Input: part model. Units: mm. Frame: model coordinates. Give positions to 0.01 mm unless a question says otherwise; leave off trailing zeros. Order: outer loops, then holes, each group sorted by start corner. A loop starts at its lowest first (then second) coordinate and runs counter-clockwise, first axis right, second up.
```python
from build123d import *

# Parameters (mm, degrees)
SKETCH2_W           = 50
SKETCH2_H           = 50
BOSS_EXTRUDE1_DEPTH = 5
SKETCH6_W           = 42.36475395
SKETCH6_H           = 2.5
CUT_EXTRUDE1_DEPTH  = 50
SKETCH9_W           = 1.188642814
SKETCH9_H           = 2.221510963
CUT_EXTRUDE3_DEPTH  = 50
FILLET2_R           = 1
FILLET3_R           = 1
SKETCH11_W          = 1.18864281
SKETCH11_H          = 2.22151096
CUT_EXTRUDE4_DEPTH  = 50
FILLET5_R           = 1
FILLET6_R           = 1
SKETCH14_W          = 3.817623025
SKETCH14_H          = 0.21818248
CUT_EXTRUDE5_DEPTH  = 50
SKETCH16_W          = 3.817623025
SKETCH16_H          = 0.211754728
CUT_EXTRUDE6_DEPTH  = 50


with BuildPart() as part:
    # Sketch2 → Boss-Extrude1 (new body)
    with BuildSketch(Plane(origin=(0, 0, 0), x_dir=(1, 0, 0), z_dir=(0, 1, 0))):
        Rectangle(SKETCH2_W, SKETCH2_H)
    extrude(amount=BOSS_EXTRUDE1_DEPTH)

    # Sketch6 → Cut-Extrude1 (cut)
    with BuildSketch(Plane(origin=(0, 0, -25), x_dir=(-1, 0, 0), z_dir=(0, 0, -1))):
        with Locations((0, 1.25)):
            Rectangle(SKETCH6_W, SKETCH6_H)
    extrude(amount=-CUT_EXTRUDE1_DEPTH, mode=Mode.SUBTRACT)

    # Sketch9 → Cut-Extrude3 (cut)
    with BuildSketch(Plane(origin=(0, 0, -25), x_dir=(-1, 0, 0), z_dir=(0, 0, -1))):
        with Locations((-21.776698382, 1.389244518)):
            Rectangle(SKETCH9_W, SKETCH9_H)
    extrude(amount=-CUT_EXTRUDE3_DEPTH, mode=Mode.SUBTRACT)

    # Fillet2
    fillet2_edges = [part.edges().sort_by_distance(p)[0] for p in [
        (22.371019789, 2.5, 0),
    ]]
    fillet(fillet2_edges, radius=FILLET2_R)

    # Fillet3
    fillet3_edges = [part.edges().sort_by_distance(p)[0] for p in [
        (22.371019789, 0.278489037, 0),
    ]]
    fillet(fillet3_edges, radius=FILLET3_R)

    # Sketch11 → Cut-Extrude4 (cut)
    with BuildSketch(Plane.XY.offset(25)):
        with Locations((-21.77669838, 1.38924452)):
            Rectangle(SKETCH11_W, SKETCH11_H)
    extrude(amount=-CUT_EXTRUDE4_DEPTH, mode=Mode.SUBTRACT)

    # Fillet5
    fillet5_edges = [part.edges().sort_by_distance(p)[0] for p in [
        (-22.371019785, 2.5, 0),
    ]]
    fillet(fillet5_edges, radius=FILLET5_R)

    # Fillet6
    fillet6_edges = [part.edges().sort_by_distance(p)[0] for p in [
        (-22.371019785, 0.27848904, 0),
    ]]
    fillet(fillet6_edges, radius=FILLET6_R)

    # Sketch14 → Cut-Extrude5 (cut)
    with BuildSketch(Plane.XY.offset(25)):
        with Locations((-23.091188487, 0.10909124)):
            Rectangle(SKETCH14_W, SKETCH14_H)
    extrude(amount=-CUT_EXTRUDE5_DEPTH, mode=Mode.SUBTRACT)

    # Sketch16 → Cut-Extrude6 (cut)
    with BuildSketch(Plane.XY.offset(25)):
        with Locations((23.091188487, 0.105877364)):
            Rectangle(SKETCH16_W, SKETCH16_H)
    extrude(amount=-CUT_EXTRUDE6_DEPTH, mode=Mode.SUBTRACT)


solid = part.part
```
1) Cut plane A-A (z = 16.5). Return the cut outline in (x, y).
2) First-contact query: P1, Ø3, axis at x = -22.5, z = -9.5, coming from the -Y side; P2, Ø13, axis at x = 9, z = -10, coming from the -Y side. Flat tips, straight axial feed; report the tip coordinate or a pass-through.
3) Pull-direction query (X, two-part tool) for faces 1 (the face through (-25, 3, 0)), 2 (the face through (0, 4, -25)), 3 (the face through (25, 3, 0)), 4 (the face through (0, 2.5, 0)); classes: pulls with the +X half, pulls with the -X half, needs draft (parallel to the pull), parting line crosses it, or undercut.
4) Cut plane B-B (x = 7.5). Return the cut outline in (y, z).
5) Line query: probe 1 along Y at (x, z) = (20, -21.5); probe 2 along Y at (x, z) = (-22, -10); probe 3 along X at (y, z) = (1.9, 17.5). Output: solid intervals per line, ascending.
Geometry says:
1. outline: (-25, 0.22) - (-21.18, 0.22) - (-21.18, 0.28) - (-21.37, 0.28) arc R1 cw to (-22.37, 1.28) - (-22.37, 1.5) arc R1 cw to (-21.37, 2.5) - (21.37, 2.5) arc R1 cw to (22.37, 1.5) - (22.37, 1.28) arc R1 cw to (21.37, 0.28) - (21.18, 0.28) - (21.18, 0.21) - (25, 0.21) - (25, 5) - (-25, 5) - close
2. P1: stops at y = 0.22
2. P2: stops at y = 2.5
3. face 1: pulls with the -X half
3. face 2: needs draft
3. face 3: pulls with the +X half
3. face 4: undercut
4. outline: (2.5, -25) - (5, -25) - (5, 25) - (2.5, 25) - close
5. probe 1: y = 2.5 to 5
5. probe 2: y = 0.22 to 0.5, 2.28 to 5
5. probe 3: x = -25 to -22.29, 22.29 to 25
